from build123d import *

# Parameters (mm, degrees)
SKETCH1_W                                         = 203.2
SKETCH1_H                                         = 101.6
BOSS_EXTRUDE1_DEPTH                               = 38.1
SKETCH2_R                                         = 76.2
CUT_EXTRUDE1_DEPTH                                = 120.811560377
SKETCH3_W                                         = 38.1
SKETCH3_H                                         = 19.05
BOSS_EXTRUDE2_DEPTH                               = 25.4
CUT_EXTRUDE2_DEPTH                                = 142.990316571
BOSS_EXTRUDE3_DEPTH                               = 38.1
BOSS_EXTRUDE4_DEPTH                               = 38.1
BOSS_EXTRUDE5_DEPTH                               = 38.1
FILLET1_R                                         = 1.27
FILLET2_R                                         = 1.27
SKETCH8_W                                         = 177.8
SKETCH8_H                                         = 152.4
CUT_EXTRUDE4_DEPTH                                = 142.990316571
FILLET3_R                                         = 1.27
CBORE_FOR_5_16_BUTTON_HEAD_CAP_SCREW1_D           = 8.4328
CBORE_FOR_5_16_BUTTON_HEAD_CAP_SCREW1_CBORE_D     = 14.68374
CBORE_FOR_5_16_BUTTON_HEAD_CAP_SCREW1_CBORE_DEPTH = 4.2164
SKETCH11_W                                        = 11.022458007
SKETCH11_H                                        = 35.608864266
BOSS_EXTRUDE6_DEPTH                               = 38.1
FILLET4_R                                         = 1.27
SKETCH15_W                                        = 13.208
SKETCH15_H                                        = 6.985
CUT_EXTRUDE6_DEPTH                                = 19.05
FILLET5_R                                         = 1.27


with BuildPart() as part:
    # Sketch1 → Boss-Extrude1 (new body)
    with BuildSketch(Plane.XY):
        Rectangle(SKETCH1_W, SKETCH1_H)
    extrude(amount=BOSS_EXTRUDE1_DEPTH)

    # Sketch2 → Cut-Extrude1 (cut, through all)
    with BuildSketch(Plane.XY.offset(38.1)):
        with Locations((0, 50.8)):
            Circle(SKETCH2_R)
    extrude(amount=-CUT_EXTRUDE1_DEPTH, mode=Mode.SUBTRACT)

    # Sketch3 → Boss-Extrude2 (add)
    with BuildSketch(Plane.ZY.offset(101.6)):
        with Locations((19.05, -41.275)):
            Rectangle(SKETCH3_W, SKETCH3_H)
    extrude(amount=BOSS_EXTRUDE2_DEPTH)

    # Sketch4 → Cut-Extrude2 (cut, through all)
    with BuildSketch(Plane.XY.offset(38.1)):
        with BuildLine():
            Line((-85.194189943, 41.275), (-92.075, 41.275))
            Line((-92.075, 41.275), (-92.075, -41.275))
            Line((-92.075, -41.275), (-36.602542053, -41.275))
            Line((-36.602542053, -41.275), (-36.602542053, -26.717930443))
            ThreePointArc((-36.602542053, -26.717930443), (-69.745040174, 0.956194004), (-85.194189943, 41.275))
        make_face()
    extrude(amount=-CUT_EXTRUDE2_DEPTH, mode=Mode.SUBTRACT)

    # Sketch5 → Boss-Extrude3 (add)
    with BuildSketch(Plane.XY.offset(38.1)):
        with BuildLine():
            Line((-62.678249532, -3.066814498), (-97.060420113, -12.27948934))
            ThreePointArc((-97.060420113, -12.27948934), (-100.94898508, -10.03442531), (-98.70392105, -6.145860343))
            Line((-98.70392105, -6.145860343), (-64.321750468, 3.066814498))
            ThreePointArc((-64.321750468, 3.066814498), (-60.433185502, 0.821750468), (-62.678249532, -3.066814498))
        make_face()
    extrude(amount=-BOSS_EXTRUDE3_DEPTH)

    # Sketch6 → Boss-Extrude4 (add)
    with BuildSketch(Plane.XY.offset(38.1)):
        with BuildLine():
            Line((-60.889539792, -1.807241683), (-89.464539792, -43.082241683))
            ThreePointArc((-89.464539792, -43.082241683), (-93.882241683, -43.885460208), (-94.685460208, -39.467758317))
            Line((-94.685460208, -39.467758317), (-66.110460208, 1.807241683))
            ThreePointArc((-66.110460208, 1.807241683), (-61.692758317, 2.610460208), (-60.889539792, -1.807241683))
        make_face()
    extrude(amount=-BOSS_EXTRUDE4_DEPTH)

    # Sketch7 → Boss-Extrude5 (add)
    with BuildSketch(Plane.XY.offset(38.1)):
        with BuildLine():
            Line((-60.325, 0), (-60.325, -43.707479127))
            ThreePointArc((-60.325, -43.707479127), (-63.5, -46.882479127), (-66.675, -43.707479127))
            Line((-66.675, -43.707479127), (-66.675, 0))
            ThreePointArc((-66.675, 0), (-63.5, 3.175), (-60.325, 0))
        make_face()
    extrude(amount=-BOSS_EXTRUDE5_DEPTH)

    # Fillet1
    fillet1_edges = [part.edges().sort_by_distance(p)[0] for p in [
        (-60.325, -41.275, 19.05),
        (-66.675, -41.275, 19.05),
        (-101.6, -31.75, 19.05),
        (-127, -31.75, 19.05),
        (-85.194189943, 41.275, 19.05),
        (-36.602542053, -26.717930443, 19.05),
        (-92.075, 41.275, 19.05),
        (-92.075, -4.369646301, 19.05),
        (-92.075, -10.943650047, 19.05),
        (-70.136622156, 1.508724326, 19.05),
        (-101.6, 50.8, 19.05),
    ]]
    fillet(fillet1_edges, radius=FILLET1_R)

    # Fillet2
    fillet2_edges = [part.edges().sort_by_distance(p)[0] for p in [
        (-92.075, -35.697093572, 19.05),
        (-66.675, -10.164017539, 19.05),
        (-60.325, -10.107060346, 19.05),
        (-71.03501409, -5.306002813, 19.05),
        (-88.213372473, -41.275, 19.05),
    ]]
    fillet(fillet2_edges, radius=FILLET2_R)

    # Sketch8 → Cut-Extrude4 (cut, through all)
    with BuildSketch(Plane.XY.offset(38.1)):
        with Locations((61.822457947, 25.4)):
            Rectangle(SKETCH8_W, SKETCH8_H)
    extrude(amount=-CUT_EXTRUDE4_DEPTH, mode=Mode.SUBTRACT)

    # Fillet3
    fillet3_edges = [part.edges().sort_by_distance(p)[0] for p in [
        (-127, -50.8, 19.05),
        (-27.077542053, -20.426727542, 19.05),
        (-27.077542053, -50.8, 19.05),
        (-36.602542053, -41.275, 19.05),
    ]]
    fillet(fillet3_edges, radius=FILLET3_R)

    # CBORE for 5/16 Button Head Cap Screw1 (through all)
    with Locations(Plane(origin=(0, -31.75, 0), x_dir=(1, 0, 0), z_dir=(0, 1, 0))):
        with Locations((-114.3, -19.05)):
            CounterBoreHole(CBORE_FOR_5_16_BUTTON_HEAD_CAP_SCREW1_D / 2, CBORE_FOR_5_16_BUTTON_HEAD_CAP_SCREW1_CBORE_D / 2, CBORE_FOR_5_16_BUTTON_HEAD_CAP_SCREW1_CBORE_DEPTH)

    # Sketch11 → Boss-Extrude6 (add)
    with BuildSketch(Plane.XY.offset(38.1)):
        with Locations((-32.588771057, -32.995567867)):
            Rectangle(SKETCH11_W, SKETCH11_H)
    extrude(amount=-BOSS_EXTRUDE6_DEPTH)

    # Fillet4
    fillet4_edges = [part.edges().sort_by_distance(p)[0] for p in [
        (-27.077542053, -15.191135734, 19.05),
        (-27.077542053, -50.8, 19.05),
    ]]
    fillet(fillet4_edges, radius=FILLET4_R)

    # Sketch15 → Cut-Extrude6 (cut)
    with BuildSketch(Plane(origin=(-27.077542053, 0, 0), x_dir=(0, 0, -1), z_dir=(1, 0, 0))):
        with Locations((-19.05, -47.3075)):
            Rectangle(SKETCH15_W, SKETCH15_H)
    extrude(amount=-CUT_EXTRUDE6_DEPTH, mode=Mode.SUBTRACT)

    # Fillet5
    fillet5_edges = [part.edges().sort_by_distance(p)[0] for p in [
        (-38.10000006, -41.275, 19.05),
        (-38.10000006, -25.993005023, 19.05),
    ]]
    fillet(fillet5_edges, radius=FILLET5_R)


solid = part.part
Check sheet for the modelled part. Datum: model origin and axes. Units: mm. A direction names the side the tool comes from. Round coordinates to 2 decimals unless told otherwise and drop trailing zeros. Loops run counter-clockwise (first coordinate to the right, second up) from the corner with the lowest first, then second, coordinate; pieces in that order, holes last. Notation, with made-up numbers: (23.25, 23) -> (60.25, 23) arc R31 ccw to (60.25, 62) -> close; hole circle Ø3 at (58, -38). An arc over 180 degrees is marked (long way). Put each result on its own line as item: value. Start each with the question number.
1. Section check C-C (y = -9.5). Enter the section's corners in (x, z), plus the area to 3 significant figures.
2. Scan lines: probe 1 along Z at (x, y) = (-114, -39); probe 2 along X at (y, z) = (-40, 19) (3 decimals); probe 3 along X at (y, z) = (-40.5, 11). Record each from-to range of solid material in increasing order.
3. Section check D-D (x = -56). Enter the section's corners in (y, z) (3 decimals), plus the area to 3 significant figures.
4. Section check B-B (z = 19.05). Give the number of separate pieces and of enclosed holes in the cut face, plus the area to 3 significant figures.
5. Draft check along X on faces 4 (the face through (-67.545, -13.024, 18.783)), 5 (the face through (-46.128, -47, 19)), 6 (the face through (-127, -41, 19)). Enter one of: +X half, -X half, draft (parallel to the pull), parting line (faces both ways), or undercut.
6. Access from +Z, -Z, +X, -X, +Y, -Y to the whole of each face (thin tool, end or side, straight path). Record for faces 1 (the face through (-107.3, -33.83, 16.84)), 2 (the face through (-36, -47, 12.446)), 3 (the face through (-81.305, -1.484, 19.317)).
7. Section check A-A (x = -114.3). Enter the section's corners in (y, z).
8. Gauge pin test, flat ends, axial feed: pin 1 (4 mm diameter, centred on y = -4.5, z = 11.5, fed in from -X); pin 2 (14.5 mm diameter, centred on x = -76, z = 25, fed in from +Y); pin 3 (17 mm diameter, centred on x = -114.3, z = 19.05, fed in from +Y); pin 4 (10 mm diameter, centred on x = -51.5, z = 16.5, fed in from +Y). Record the tip position at first contact, or that the pin passes through.
Findings:
1. outline: (-101.6, 0) -> (-86.69, 0) -> (-86.69, 38.1) -> (-101.6, 38.1) -> close; (-73.94, 0) -> (-46.59, 0) -> (-46.59, 38.1) -> (-73.94, 38.1) -> close
1. area: 1,610 mm^2
2. probe 1: z = 0 to 14.84, 23.26 to 38.1
2. probe 2: x = -127 to -118.516, -110.084 to -87.059, -66.675 to -60.325, -38.1 to -27.078
2. probe 3: x = -127 to -86.96, -66.78 to -60.22, -38.2 to -27.08
3. outline: (-50.8, 0) -> (-41.275, 0) -> (-41.275, 38.1) -> (-50.8, 38.1) -> close; (-14.106, 0) -> (-0.876, 0) -> (-0.876, 38.1) -> (-14.106, 38.1) -> close
3. area: 867 mm^2
4. separate pieces: 2
4. enclosed holes: 4
4. area: 3,590 mm^2
5. face 4: undercut
5. face 5: +X half
5. face 6: -X half
6. face 1: +Y
6. face 2: +X, -Y
6. face 3: +Z, -Z
7. outline: (-50.8, 0) -> (-31.75, 0) -> (-31.75, 11.71) -> (-35.97, 11.71) -> (-35.97, 14.83) -> (-50.8, 14.83) -> close; (-50.8, 23.27) -> (-35.97, 23.27) -> (-35.97, 26.39) -> (-31.75, 26.39) -> (-31.75, 38.1) -> (-50.8, 38.1) -> close
8. pin 1: stops at x = -101.6
8. pin 2: stops at y = 50.8
8. pin 3: stops at y = -31.75
8. pin 4: stops at y = -0.33
